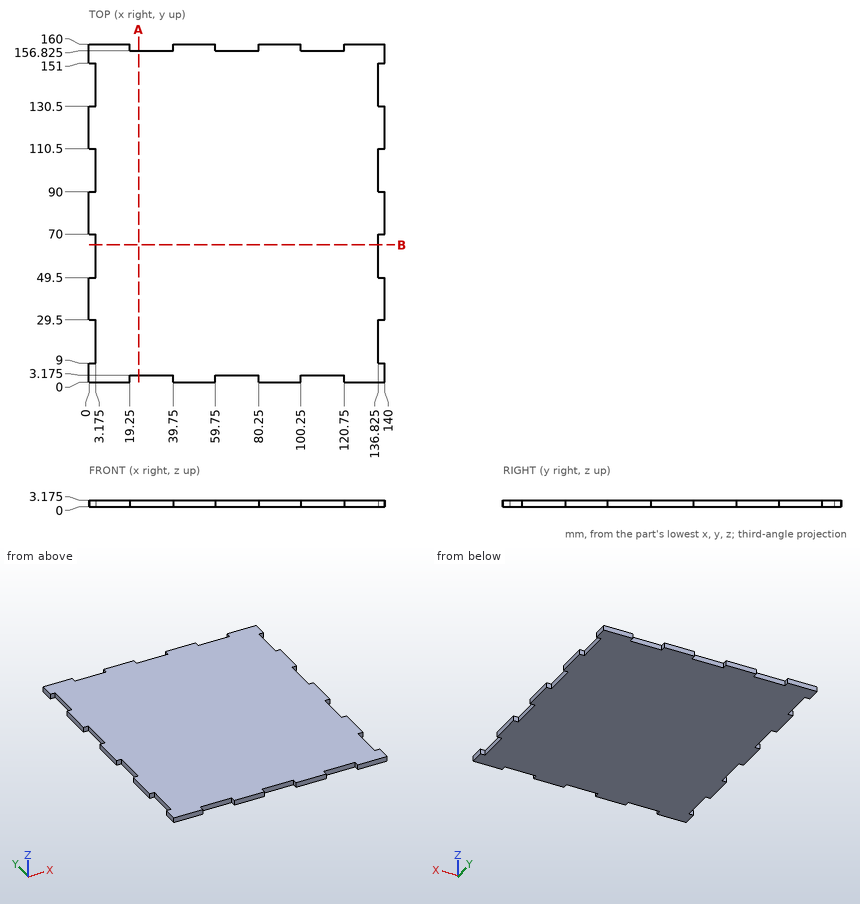
Drawing for the job (mm, zero at the part's lowest x, y, z). Coordinates: 2 decimals unless noted, no trailing zeros. Loops run counter-clockwise (first coordinate to the right, second up) from the corner with the lowest first, then second, coordinate; pieces in that order, holes last. Notation, with made-up numbers: (-24, -2) - (17, -2) arc R9 cw to (17, 15) - close; hole circle Ø6 at (68, 52.5). An arc over 180 degrees is marked (long way). Return JSON: item names as keys, results as strings.
1. Probe L1, parallel to X at y = 92.5, z = 0.2 (3 decimals); L2, parallel to Y at x = 77, z = 0.2 (3 decimals). List the from-to ranges inside material, lowest first. Write a range as from..to.
Result:
{"L1": "x = 3.175..136.825", "L2": "y = 3.175..156.825"}
2. Drop a flat-ended pin along its axis: pin 1 (1.6 mm diameter, centred on y = 141.5, z = 2, fed in from -X) (3 decimals). Give the stop position or say it passes through.
Result:
{"pin 1": "stops at x = 3.175"}
3. Band-saw the part on B-B (y = 65). Give the cut face in (x, z) (3 decimals).
Result:
{"outline": "(3.175, 0) - (136.825, 0) - (136.825, 3.175) - (3.175, 3.175) - close"}
4. Band-saw the part on A-A (x = 23.5). Give the cut face in (y, z) (3 decimals), and give its area (3 significant figures).
Result:
{"outline": "(3.175, 0) - (156.825, 0) - (156.825, 3.175) - (3.175, 3.175) - close", "area": "488 mm2"}
